The model under review builds one solid part; all positions refer to its coordinate system, in mm. A direction names the side the tool comes from. Give positions to 0.01 mm unless a question says otherwise; leave off trailing zeros. Write each loop counter-clockwise with the first axis right and the second up, starting at its lowest first coordinate (ties: lowest second). Pieces come first, ordered by that corner, then holes. Notation, with made-up numbers: (-13, 68.25) - (23, 68.25) arc R20 cw to (23, 101.25) - close; hole circle Ø10 at (89, 85.25). An arc over 180 degrees is marked (long way). Write item = value, one per line.
```python
from build123d import *

# Parameters (mm, degrees)
BOSS_EXTRUDE1_DEPTH = 10
BOSS_EXTRUDE3_START = -10
SKETCH2_W           = 25.4
SKETCH2_H           = 40
BOSS_EXTRUDE3_DEPTH = 17
FILLET2_R           = 5


with BuildPart() as part:
    # Sketch1 → Boss-Extrude1 (new body)
    with BuildSketch(Plane(origin=(0, 0, 0), x_dir=(1, 0, 0), z_dir=(0, 1, 0))):
        with BuildLine():
            Line((-40.682943279, 44.876700425), (-52.117056721, 44.876700425))
            ThreePointArc((-52.117056721, 44.876700425), (-70.45991945, 29.48934494), (-58.497022921, 8.75))
            ThreePointArc((-58.497022921, 8.75), (-70.45991945, -11.98934494), (-52.117056721, -27.376700425))
            Line((-52.117056721, -27.376700425), (-40.682943279, -27.376700425))
            Line((-40.682943279, -27.376700425), (-16.783731474, -27.376700425))
            ThreePointArc((-16.783731474, -27.376700425), (-9.130062827, -28.899109774), (-2.64159585, -33.234564801))
            Line((-2.64159585, -33.234564801), (3.142675397, -39.018836048))
            ThreePointArc((3.142675397, -39.018836048), (9.631142374, -43.354291075), (17.284811021, -44.876700425))
            Line((17.284811021, -44.876700425), (40.682943279, -44.876700425))
            Line((40.682943279, -44.876700425), (52.117056721, -44.876700425))
            ThreePointArc((52.117056721, -44.876700425), (70.45991945, -29.48934494), (58.497022921, -8.75))
            ThreePointArc((58.497022921, -8.75), (70.45991945, 11.98934494), (52.117056721, 27.376700425))
            Line((52.117056721, 27.376700425), (40.682943279, 27.376700425))
            Line((40.682943279, 27.376700425), (17.119939677, 27.376700425))
            ThreePointArc((17.119939677, 27.376700425), (9.596852719, 28.845560076), (3.17880165, 33.036384162))
            Line((3.17880165, 33.036384162), (-3.17880165, 39.217016687))
            ThreePointArc((-3.17880165, 39.217016687), (-9.596852719, 43.407840773), (-17.119939677, 44.876700425))
            Line((-17.119939677, 44.876700425), (-40.682943279, 44.876700425))
        make_face()
        with BuildLine():
            Line((-40.682943279, 10), (-52.117056721, 10))
            ThreePointArc((-52.117056721, 10), (-68.367056721, 26.25), (-52.117056721, 42.5))
            Line((-52.117056721, 42.5), (-40.682943279, 42.5))
            ThreePointArc((-40.682943279, 42.5), (-24.432943279, 26.25), (-40.682943279, 10))
        make_face(mode=Mode.SUBTRACT)
        with BuildLine():
            Line((-40.682943279, 7.5), (-52.117056721, 7.5))
            ThreePointArc((-52.117056721, 7.5), (-68.367056721, -8.75), (-52.117056721, -25))
            Line((-52.117056721, -25), (-40.682943279, -25))
            ThreePointArc((-40.682943279, -25), (-24.432943279, -8.75), (-40.682943279, 7.5))
        make_face(mode=Mode.SUBTRACT)
        with BuildLine():
            Line((40.682943279, -10), (52.117056721, -10))
            ThreePointArc((52.117056721, -10), (68.367056721, -26.25), (52.117056721, -42.5))
            Line((52.117056721, -42.5), (40.682943279, -42.5))
            ThreePointArc((40.682943279, -42.5), (24.432943279, -26.25), (40.682943279, -10))
        make_face(mode=Mode.SUBTRACT)
        with BuildLine():
            Line((40.682943279, -7.5), (52.117056721, -7.5))
            ThreePointArc((52.117056721, -7.5), (68.367056721, 8.75), (52.117056721, 25))
            Line((52.117056721, 25), (40.682943279, 25))
            ThreePointArc((40.682943279, 25), (24.432943279, 8.75), (40.682943279, -7.5))
        make_face(mode=Mode.SUBTRACT)
    extrude(amount=BOSS_EXTRUDE1_DEPTH)

    # Sketch2 → Boss-Extrude3 (add)
    with BuildSketch(Plane(origin=(0, 10, 0), x_dir=(1, 0, 0), z_dir=(0, 1, 0)).offset(BOSS_EXTRUDE3_START)):
        Rectangle(SKETCH2_W, SKETCH2_H)
    extrude(amount=-BOSS_EXTRUDE3_DEPTH)

    # Fillet2
    fillet2_edges = [part.edges().sort_by_distance(p)[0] for p in [
        (-12.7, 0, 0),
        (0, 0, 20),
        (12.7, 0, 0),
        (0, 0, -20),
    ]]
    fillet(fillet2_edges, radius=FILLET2_R)


solid = part.part
```
1. For line 1 (X direction, y = 2.5, z = -13.5); line 2 (X direction, y = 5.75, z = -17); line 3 (Z direction, x = 34.5, y = 7.75), list the stretches that pass through material, from the lowest coordinate up. Write a range as from..to.
Findings below:
line_1 = -65.7..-62.19, -30.61..25.14, 67.66..70.13
line_2 = -68.28..-65.48, -27.32..26.68, 66.12..68.82
line_3 = -27.38..-23.78, 6.28..11.22, 41.28..44.88
2. Take a section at D-D on y = -8.5. Give the boundary of the cut face in (x, z).
Findings below:
outline = (-12.7, -20) - (12.7, -20) - (12.7, 20) - (-12.7, 20) - close
3. Draft analysis for pull direction X (two halves, no side actions). For faces 1 (the flat face through (46, 5, -25)), 2 (the flat face through (-21, 0, 0)), 3 (the cylindrical face through (14.2, -1.43, -0.35)), state which applies: +X half, -X half, draft (parallel to the pull), parting line (faces both ways), or undercut.
Findings below:
face_1 = undercut
face_2 = draft
face_3 = +X half
4. Insertion check: P1, Ø13, axis at y = -11, z = -9, coming from the +X side; P2, Ø8, axis at x = 18.5, z = -25.5, coming from the -Y side; P3, Ø12, axis at y = -4, z = -2, coming from the +X side. Each pin has a flat end and moves straight along its axis. Give the tip position at first contact, or say it passes through.
Findings below:
P1 = 12.73
P2 = -0.5
P3 = 70.6
5. Machinability: for faces 4 (the cylindrical face through (9.5, 4.9, 43.3)), 5 (the cylindrical face through (24.437, 4.93, -9.107)), 6 (the flat face through (-12.7, -11, 0)), which of the approach directions +Z, -Z, +X, -X, +Y, -Y give a long, thin tool a straight path to every point of the face, cutting with its end or side? Answer none if there is none.
Findings below:
face_4 = +Z, -X, +Y, -Y
face_5 = +Y, -Y
face_6 = +Z, -Z, -X, -Y
6. Take a section at C-C on y = 7. Count the separate pieces of the cut face and the enclosed holes in it, and give its area (3 significant figures).
Findings below:
separate_pieces = 1
enclosed_holes = 4
area = 4,880 mm²
7. Take a section at A-A on x = -38.5. Give the boundary of the cut face in (y, z).
Findings below:
outline = (0, -44.88) - (10, -44.88) - (10, -42.35) - (0, -42.35) - close; (0, -10.15) - (10, -10.15) - (10, -7.35) - (0, -7.35) - close; (0, 24.85) - (10, 24.85) - (10, 27.38) - (0, 27.38) - close
8. Take a section at B-B on z = 5.5. Give the boundary of the cut face in (x, y), and give its area (3 significant figures).
Findings below:
outline = (-70.46, 0) - (-68.04, 0) - (-68.04, 10) - (-70.46, 10) - close; (-24.76, 0) - (-17.7, 0) arc R5 cw to (-12.7, -5) - (-12.7, -17) - (12.7, -17) - (12.7, -5) arc R5 cw to (17.7, 0) - (32.87, 0) - (32.87, 10) - (-24.76, 10) - close; (59.93, 0) - (64.11, 0) - (64.11, 10) - (59.93, 10) - close
area = 1,080 mm²
